Work out the finished part from the listing and answer in its coordinate system (mm). Give positions to 0.01 mm unless a question says otherwise; leave off trailing zeros. Loops run counter-clockwise (first coordinate to the right, second up) from the corner with the lowest first, then second, coordinate; pieces in that order, holes last. Notation, with made-up numbers: (82.25, 41.25) -> (94.25, 41.25) arc R11 ccw to (94.25, 53.25) -> close; hole circle Ø10 at (45, 68). An arc over 180 degrees is marked (long way). Answer as CSV lines item,"result". Start each with the question number.
1. A flat-ended cylindrical pin translates along its axis: pin 1 Ø2 at (x, y) = (2, 2) entering from +Z. Find the tip coordinate at first contact, or state that the pin passes through.
2. Find section C-C, the plane x = 3.66. Give the vertices of the cut face in (y, z).
3. Find section D-D, the plane y = 4.75. Count the separate pieces of the cut face and the enclosed holes in it, and give its area (3 significant figures).
4. Find section A-A, the plane y = -1.75. Give the vertices of the cut face in (x, z).
5. Determine the mould class of faces 1 (the face through (0, 4, -1)), 2 (the face through (4, 6, -0.75)) for opening direction Z: +Z half, -Z half, draft (parallel to the pull), parting line (faces both ways), or undercut.
6. Find the intervals of material crossed by line 1 along Z through (x, y) = (5.75, 6.5); line 2 along Y through (x, z) = (13.25, -0.2), in increasing order.
from build123d import *

# Parameters (mm, degrees)
SKETCH1_W           = 16
SKETCH1_H           = 2.5
BOSS_EXTRUDE1_DEPTH = 8.5
SKETCH2_W           = 1
SKETCH2_H           = 1
CUT_EXTRUDE1_DEPTH  = 5
CHAMFER1_SIZE       = 0.5
SKETCH3_R           = 0.25
BOSS_EXTRUDE2_DEPTH = 6.5


with BuildPart() as part:
    # Sketch1 → Boss-Extrude1 (new body)
    with BuildSketch(Plane(origin=(0, 0, 0), x_dir=(1, 0, 0), z_dir=(0, 1, 0))):
        with Locations((8, 1.25)):
            Rectangle(SKETCH1_W, SKETCH1_H)
    extrude(amount=BOSS_EXTRUDE1_DEPTH)

    # Sketch2 → Cut-Extrude1 (cut)
    with BuildSketch(Plane(origin=(0, 8.5, 0), x_dir=(1, 0, 0), z_dir=(0, 1, 0))):
        with Locations((1.5, 1.25)):
            Rectangle(SKETCH2_W, SKETCH2_H)
        with Locations((3.66, 1.25)):
            Rectangle(SKETCH2_W, SKETCH2_H)
        with Locations((5.82, 1.25)):
            Rectangle(SKETCH2_W, SKETCH2_H)
        with Locations((7.98, 1.25)):
            Rectangle(SKETCH2_W, SKETCH2_H)
        with Locations((10.14, 1.25)):
            Rectangle(SKETCH2_W, SKETCH2_H)
        with Locations((12.3, 1.25)):
            Rectangle(SKETCH2_W, SKETCH2_H)
        with Locations((14.46, 1.25)):
            Rectangle(SKETCH2_W, SKETCH2_H)
    extrude(amount=-CUT_EXTRUDE1_DEPTH, mode=Mode.SUBTRACT)

    # Chamfer1
    chamfer1_edges = [part.edges().sort_by_distance(p)[0] for p in [
        (1, 8.5, -1.25),
        (1.5, 8.5, -0.75),
        (2, 8.5, -1.25),
        (1.5, 8.5, -1.75),
        (3.16, 8.5, -1.25),
        (3.66, 8.5, -0.75),
        (4.16, 8.5, -1.25),
        (3.66, 8.5, -1.75),
        (5.32, 8.5, -1.25),
        (5.82, 8.5, -0.75),
        (6.32, 8.5, -1.25),
        (5.82, 8.5, -1.75),
        (7.48, 8.5, -1.25),
        (7.98, 8.5, -0.75),
        (8.48, 8.5, -1.25),
        (7.98, 8.5, -1.75),
        (9.64, 8.5, -1.25),
        (10.14, 8.5, -0.75),
        (10.64, 8.5, -1.25),
        (10.14, 8.5, -1.75),
        (11.8, 8.5, -1.25),
        (12.3, 8.5, -0.75),
        (12.8, 8.5, -1.25),
        (12.3, 8.5, -1.75),
        (13.96, 8.5, -1.25),
        (14.46, 8.5, -0.75),
        (14.96, 8.5, -1.25),
        (14.46, 8.5, -1.75),
    ]]
    chamfer(chamfer1_edges, length=CHAMFER1_SIZE)

    # Sketch3 → Boss-Extrude2 (add)
    with BuildSketch(Plane(origin=(0, 3.5, 0), x_dir=(1, 0, 0), z_dir=(0, 1, 0))):
        with Locations((1.5, 1.25)):
            Circle(SKETCH3_R)
        with Locations((3.66, 1.25)):
            Circle(SKETCH3_R)
        with Locations((5.82, 1.25)):
            Circle(SKETCH3_R)
        with Locations((7.98, 1.25)):
            Circle(SKETCH3_R)
        with Locations((10.14, 1.25)):
            Circle(SKETCH3_R)
        with Locations((12.3, 1.25)):
            Circle(SKETCH3_R)
        with Locations((14.46, 1.25)):
            Circle(SKETCH3_R)
    extrude(amount=-BOSS_EXTRUDE2_DEPTH)


solid = part.part
Resolved:
1,pin 1,"stops at z = 0"
2,outline,"(-3, -1.5) -> (0, -1.5) -> (0, -2.5) -> (8.5, -2.5) -> (8.5, -2.25) -> (8, -1.75) -> (3.5, -1.75) -> (3.5, -0.75) -> (8, -0.75) -> (8.5, -0.25) -> (8.5, 0) -> (0, 0) -> (0, -1) -> (-3, -1) -> close"
3,separate pieces,"1"
3,enclosed holes,"7"
3,area,"33.0 mm^2"
4,outline,"circle Ø0.5 at (1.5, -1.25); circle Ø0.5 at (3.66, -1.25); circle Ø0.5 at (5.82, -1.25); circle Ø0.5 at (7.98, -1.25); circle Ø0.5 at (10.14, -1.25); circle Ø0.5 at (12.3, -1.25); circle Ø0.5 at (14.46, -1.25)"
5,face 1,"draft"
5,face 2,"undercut"
6,line 1,"z = -2.5 to -1.75, -0.75 to 0"
6,line 2,"y = 0 to 8.5"
